from build123d import *

# Parameters (mm, degrees)
SKETCH1_W                         = 35
SKETCH1_H                         = 72.57
BOSS_EXTRUDE1_DEPTH               = 22
SKETCH2_W                         = 58
SKETCH2_H                         = 22
BOSS_EXTRUDE2_DEPTH               = 29.71
SKETCH3_R                         = 9.175
BOSS_EXTRUDE3_DEPTH               = 50.11
M4_CLEARANCE_HOLE1_D              = 4.5
PIPE_TAP_DRILL_FOR_1_4_TAP1_D     = 11.1252
PIPE_TAP_DRILL_FOR_1_4_TAP1_DEPTH = 15
PIPE_TAP_DRILL_FOR_1_4_TAP1_TIP   = 3.342347279
PIPE_TAP_DRILL_FOR_1_4_TAP2_D     = 11.1252
PIPE_TAP_DRILL_FOR_1_4_TAP2_DEPTH = 15
PIPE_TAP_DRILL_FOR_1_4_TAP2_TIP   = 3.342347279


with BuildPart() as part:
    # Sketch1 → Boss-Extrude1 (new body)
    with BuildSketch(Plane.XY):
        Rectangle(SKETCH1_W, SKETCH1_H)
    extrude(amount=BOSS_EXTRUDE1_DEPTH)

    # Sketch2 → Boss-Extrude2 (add)
    with BuildSketch(Plane(origin=(0, 36.285, 0), x_dir=(1, 0, 0), z_dir=(0, 1, 0))):
        with Locations((-17.6, -11)):
            Rectangle(SKETCH2_W, SKETCH2_H)
    extrude(amount=BOSS_EXTRUDE2_DEPTH)

    # Sketch3 → Boss-Extrude3 (add)
    with BuildSketch(Plane.XZ.offset(-36.285)):
        with Locations(Location((-37.425, 11, 0), (0, 0, 270))):
            Circle(SKETCH3_R)
    extrude(amount=-BOSS_EXTRUDE3_DEPTH)

    # M4 Clearance Hole1 (through all)
    with Locations(Plane.XY.offset(22)):
        with Locations((-8.8, 3.415), (-8.8, -21.285)):
            Hole(M4_CLEARANCE_HOLE1_D / 2)

    # Pipe Tap Drill for 1_4 Tap1
    with Locations(Plane.ZY.offset(17.5)):
        with Locations((11, -7.985)):
            Hole(PIPE_TAP_DRILL_FOR_1_4_TAP1_D / 2, depth=PIPE_TAP_DRILL_FOR_1_4_TAP1_DEPTH)
            with Locations((0, 0, -(PIPE_TAP_DRILL_FOR_1_4_TAP1_DEPTH + PIPE_TAP_DRILL_FOR_1_4_TAP1_TIP / 2))):  # 118° drill point
                Cone(0, PIPE_TAP_DRILL_FOR_1_4_TAP1_D / 2, PIPE_TAP_DRILL_FOR_1_4_TAP1_TIP, mode=Mode.SUBTRACT)

    # Pipe Tap Drill for 1_4 Tap2
    with Locations(Plane(origin=(17.5, 0, 0), x_dir=(0, 0, -1), z_dir=(1, 0, 0))):
        with Locations((-11, 3.315), (-11, -19.685)):
            Hole(PIPE_TAP_DRILL_FOR_1_4_TAP2_D / 2, depth=PIPE_TAP_DRILL_FOR_1_4_TAP2_DEPTH)
            with Locations((0, 0, -(PIPE_TAP_DRILL_FOR_1_4_TAP2_DEPTH + PIPE_TAP_DRILL_FOR_1_4_TAP2_TIP / 2))):  # 118° drill point
                Cone(0, PIPE_TAP_DRILL_FOR_1_4_TAP2_D / 2, PIPE_TAP_DRILL_FOR_1_4_TAP2_TIP, mode=Mode.SUBTRACT)


solid = part.part
Could you check a few things on this model? Use its own coordinates, in mm. A direction names the side the tool comes from. Round coordinates to 2 decimals unless told otherwise and drop trailing zeros. Write each loop counter-clockwise with the first axis right and the second up, starting at its lowest first coordinate (ties: lowest second). Pieces come first, ordered by that corner, then holes. Notation, with made-up numbers: (72.25, 37) -> (107.25, 37) arc R33 ccw to (107.25, 71) -> close; hole circle Ø10 at (32, 89). An arc over 180 degrees is marked (long way). Use a Markdown table: item, result.
1. We'd pull the mould along X, two halves only. Please class faces 1 (the face through (-10.01, -19.39, 10.85)), 2 (the face through (0.26, -8.57, 10.23)), 3 (the face through (-0.26, 3.97, 11.71)): +X half, -X half, draft (parallel to the pull), parting line (faces both ways), or undercut.
Answer key:
| item | result |
|---|---|
| face 1 | undercut |
| face 2 | -X half |
| face 3 | +X half |
2. If we section it at D-D (x = 6): List the corners of the cut face in (y, z) for me (3 decimals), then the cut area to 3 significant figures.
Answer key:
| item | result |
|---|---|
| outline | (-36.285, 0) -> (65.995, 0) -> (65.995, 22) -> (-36.285, 22) -> close; hole circle Ø11.125 at (-19.685, 11); hole circle Ø11.125 at (3.315, 11) |
| area | 2,060 mm^2 |
3. If we section it at C-C (y = 48.5): List the corners of the cut face in (x, z) for me, then the cut area to 3 significant figures.
Answer key:
| item | result |
|---|---|
| outline | (-46.6, 0) -> (11.4, 0) -> (11.4, 22) -> (-46.6, 22) -> close |
| area | 1,280 mm^2 |
4. Which directions (+Z, -Z, +X, -X, +Y, -Y) give clear straight access to the entire face, cutting with the end or side of a thin tool? Please do faces 4 (the face through (11.4, 51, 11)), 5 (the face through (-9.9, -6.3, 5.7)), 6 (the face through (-43.01, 76.05, 18.28)).
Answer key:
| item | result |
|---|---|
| face 4 | +Z, -Z, +X, +Y |
| face 5 | -X |
| face 6 | +Y |
5. If we section it at A-A (x = -8.8): List the corners of the cut face in (y, z) for me (3 decimals), then the cut area to 3 significant figures.
Answer key:
| item | result |
|---|---|
| outline | (-36.285, 0) -> (-23.535, 0) -> (-23.535, 22) -> (-36.285, 22) -> close; (-19.035, 0) -> (1.165, 0) -> (1.165, 22) -> (-19.035, 22) -> close; (5.665, 0) -> (65.995, 0) -> (65.995, 22) -> (5.665, 22) -> close; hole circle Ø11.125 at (-7.985, 11) |
| area | 1,950 mm^2 |
6. Please list where these lines run through material, in increasing order: probe 1 along Y at (x, z) = (9.25, 11) (3 decimals); probe 2 along Y at (x, z) = (12.25, 11) (3 decimals); probe 3 along Y at (x, z) = (-8.8, 13) (3 decimals).
Answer key:
| item | result |
|---|---|
| probe 1 | y = -36.285 to -25.248, -14.122 to -2.248, 8.878 to 65.995 |
| probe 2 | y = -36.285 to -25.248, -14.122 to -2.248, 8.878 to 36.285 |
| probe 3 | y = -36.285 to -23.535, -19.035 to -13.176, -2.794 to 1.165, 5.665 to 65.995 |
7. For pin 1 Ø6.5 at (x, z) = (-9, 15.5) entering from +Y (3 decimals); pin 2 Ø7 at (x, y) = (-8.8, -21.285) entering from -Z; pin 3 Ø13 at (y, z) = (-7.985, 11) entering from -X; pin 4 Ø1.5 at (y, z) = (56, 9) entering from +X, each with a flat end and sliding along its axis, tell me the tip position at first contact or that it passes through.
Answer key:
| item | result |
|---|---|
| pin 1 | stops at y = 65.995 |
| pin 2 | stops at z = 0 |
| pin 3 | stops at x = -17.5 |
| pin 4 | stops at x = 11.4 |
8. If we section it at B-B (z = 4): List the corners of the cut face in (x, y) for me (3 decimals).
Answer key:
| item | result |
|---|---|
| outline | (-46.6, 36.285) -> (-17.5, 36.285) -> (-17.5, -36.285) -> (17.5, -36.285) -> (17.5, 36.285) -> (11.4, 36.285) -> (11.4, 65.995) -> (-31.494, 65.995) -> (-31.494, 86.395) -> (-43.356, 86.395) -> (-43.356, 65.995) -> (-46.6, 65.995) -> close; hole circle Ø4.5 at (-8.8, -21.285); hole circle Ø4.5 at (-8.8, 3.415) |
